Geometry: see drawing. Coordinates: mm, zero at the bounding-box minimum. Round coordinates to 2 decimals unless told otherwise and drop trailing zeros. Write each loop counter-clockwise with the first axis right and the second up, starting at its lowest first coordinate (ties: lowest second). Pieces come first, ordered by that corner, then holes.
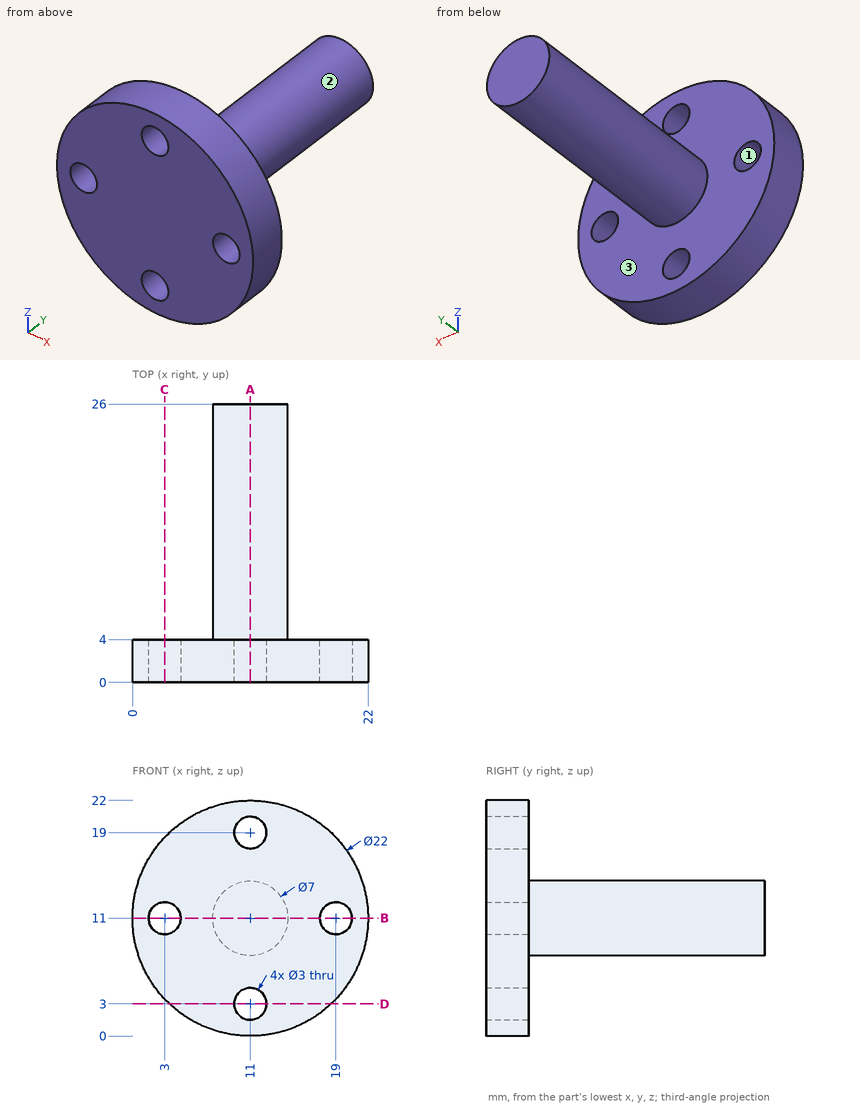
1) Material intervals for line 1 (Z direction, x = 11, y = 2.9); line 2 (Y direction, x = 7.75, z = 20); line 3 (X direction, y = 1.5, z = 19), sorted ascending.
Taken from the geometry:
line 1: z = 0 to 1.5, 4.5 to 17.5, 20.5 to 22
line 2: y = 0 to 4
line 3: x = 3.45 to 9.5, 12.5 to 18.55
2) Pull-direction query (X, two-part tool) for the marked faces 1, 2 and 3; classes: released by +X, released by -X, zero draft, split by the parting line, or undercut.
Taken from the geometry:
face 1: undercut
face 2: split by the parting line
face 3: zero draft
3) Section query A-A on x = 11. Return the cut outline in (y, z), then the cut area to 3 significant figures.
Taken from the geometry:
outline: (0, 0) - (4, 0) - (4, 1.5) - (0, 1.5) - close; (0, 4.5) - (4, 4.5) - (4, 7.5) - (26, 7.5) - (26, 14.5) - (4, 14.5) - (4, 17.5) - (0, 17.5) - close; (0, 20.5) - (4, 20.5) - (4, 22) - (0, 22) - close
area: 218 mm2
4) Section query C-C on x = 3. Return the cut outline in (y, z).
Taken from the geometry:
outline: (0, 3.45) - (4, 3.45) - (4, 9.5) - (0, 9.5) - close; (0, 12.5) - (4, 12.5) - (4, 18.55) - (0, 18.55) - close
5) Section query B-B on z = 11. Return the cut outline in (x, y).
Taken from the geometry:
outline: (0, 0) - (1.5, 0) - (1.5, 4) - (0, 4) - close; (4.5, 0) - (17.5, 0) - (17.5, 4) - (14.5, 4) - (14.5, 26) - (7.5, 26) - (7.5, 4) - (4.5, 4) - close; (20.5, 0) - (22, 0) - (22, 4) - (20.5, 4) - close
6) Section query D-D on z = 3. Return the cut outline in (x, y).
Taken from the geometry:
outline: (3.45, 0) - (9.5, 0) - (9.5, 4) - (3.45, 4) - close; (12.5, 0) - (18.55, 0) - (18.55, 4) - (12.5, 4) - close
7) Contact query for flat-ended pins moving along their axis: P1, Ø6, axis at x = 19, y = 12.5, coming from the +Z side; P2, Ø4, axis at x = 10, z = 10, coming from the -Y side; P3, Ø1.5, axis at x = 9, z = 4.5, coming from the +Y side; P4, Ø4, axis at y = 15, z = 15, coming from the +X side. Output: stop coordinate, or through.
Taken from the geometry:
P1: passes through
P2: stops at y = 0
P3: stops at y = 4
P4: stops at x = 13.87
